Print and shaded views of the part. All mm, measured from the part's lowest x, y and z. A direction names the side the tool comes from. Coordinates: 2 decimals unless noted, no trailing zeros. Loops run counter-clockwise (first coordinate to the right, second up) from the corner with the lowest first, then second, coordinate; pieces in that order, holes last.
1) Pin check, flat tips, straight feed: pin 1 Ø3 at (x, y) = (23.5, 14.5) entering from +Z; pin 2 Ø5.5 at (x, z) = (27, 73) entering from +Y; pin 3 Ø3 at (x, z) = (17, 17) entering from +Y. Stop position of each tip, or through.
2) Saw through at B-B, the plane x = 15. Write the cut outline in (y, z), and give its area (3 significant figures).
3) Saw through at D-D, the plane y = 21.25. Write the cut outline in (x, z).
4) Which spindle directions (+Z, -Z, +X, -X, +Y, -Y) get a long thin tool onto all of the face, cutting with end or side? Do the marked faces 1 and 2. Say none if no direction does.
5) Wall check: line 1 along Z through (x, y) = (1, 17); line 2 along Y through (x, z) = (22, 71); line 3 along X through (y, z) = (18.5, 8.5). Give the ranges that are in metal, low to high.
6) Saw through at A-A, the plane y = 5. Write the cut outline in (x, z), and give its area (3 significant figures).
7) Saw through at C-C, the plane z = 7. Write the cut outline in (x, y), and give its area (3 significant figures).
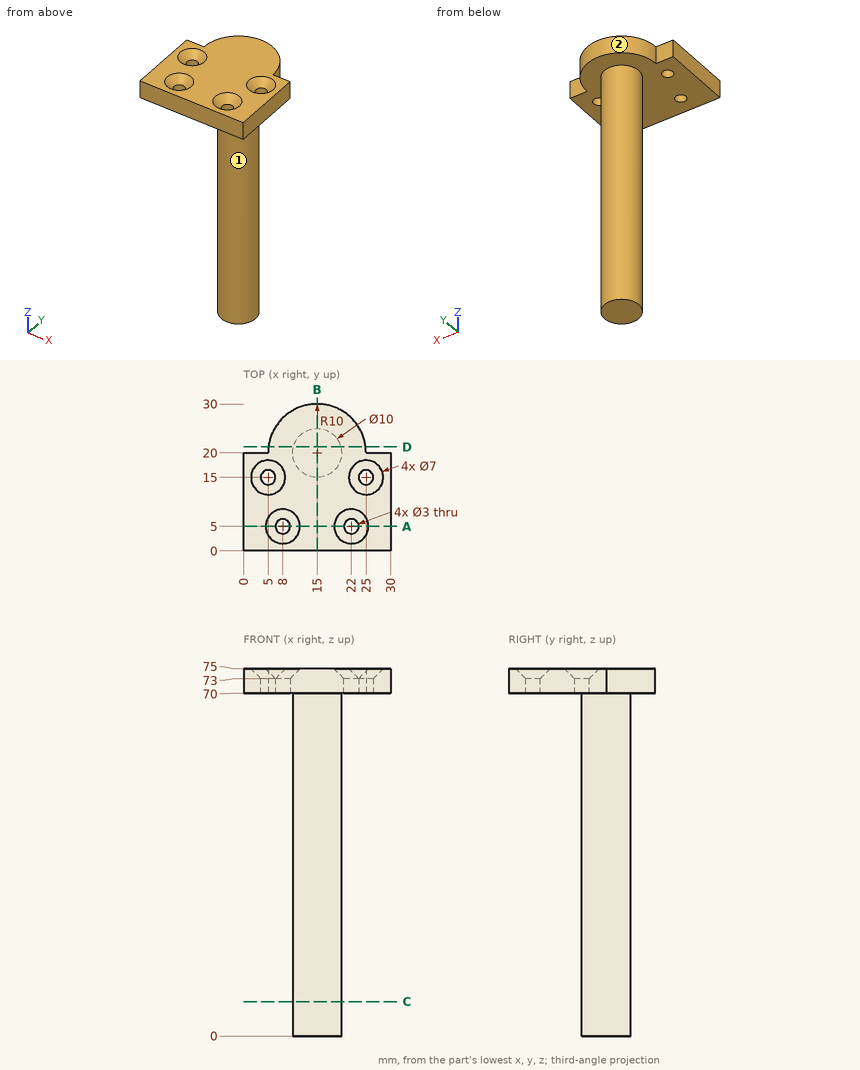
Data:
1. pin 1: stops at z = 74.58
1. pin 2: stops at y = 23.8
1. pin 3: stops at y = 24.97
2. outline: (0, 70) - (15, 70) - (15, 0) - (25, 0) - (25, 70) - (30, 70) - (30, 75) - (0, 75) - close
2. area: 850 mm2
3. outline: (5.08, 70) - (10.16, 70) - (10.16, 0) - (19.84, 0) - (19.84, 70) - (24.92, 70) - (24.92, 75) - (5.08, 75) - close
4. face 1: -Z
4. face 2: +Z, -Z, +Y
5. line 1: z = 70 to 75
5. line 2: y = 0 to 3.5, 6.5 to 27.14
5. line 3: x = 10.23 to 19.77
6. outline: (0, 70) - (6.5, 70) - (6.5, 73) - (4.5, 75) - (0, 75) - close; (9.5, 70) - (20.5, 70) - (20.5, 73) - (18.5, 75) - (11.5, 75) - (9.5, 73) - close; (23.5, 70) - (30, 70) - (30, 75) - (25.5, 75) - (23.5, 73) - close
6. area: 112 mm2
7. outline: circle Ø10 at (15, 20)
7. area: 78.5 mm2
